Autodesk Inventor part; units mm, degrees
ref_plane "YZ Plane" through (0, 0, 0) normal (1, 0, 0) x (0, 1, 0)
ref_plane "XZ Plane" through (0, 0, 0) normal (0, 1, 0) x (-1, 0, 0)
ref_plane "XY Plane" through (0, 0, 0) normal (0, 0, 1) x (1, 0, 0)
sketch "Esboço1" plane through (0, 0, 0) normal (0, 0, 1) x (1, 0, 0)
  line L0 (0, 0) -> (110, 0)
  line L1 (110, 0) -> (110, 15)
  line L2 (110, 15) -> (0, 15)
  line L3 (0, 15) -> (0, 0)
  dimension "d0" = 110
  dimension "d1" = 15
extrude "Extrusão1" add sketch "Esboço1" along normal blind 15
chamfer "Chanfro1" distance 10 distance2 32 1 edges at (110, 15, 7.5) measured on face at (110, 5, 5)
sketch "Esboço2" plane through (0, 0, 0) normal (0, -1, 0) x (1, 0, 0)
  line L0 (0, 15) -> (110, 15)
  line L1 (0, 0) -> (0, 15)
  point P0 (13, 7.5)
  point P1 (66, 7.5)
  dimension "d7" = 7.5
  dimension "d8" = 13
  dimension "d25" = 53
hole "Furo1" at (13, 0, 7.5) at (66, 0, 7.5) direction (0, 1, 0) diameter 8.376 end through all
properties part number "Garra2"
Can you work these out from the model? Positions are in its coordinate system, mm. Coordinates: 2 decimals unless noted, no trailing zeros. Write each loop counter-clockwise with the first axis right and the second up, starting at its lowest first coordinate (ties: lowest second). Pieces come first, ordered by that corner, then holes.
Q1. If we mould it in two halves opening along Z, with no side actions, what happens to faces 1 (the face through (0, 8, 7)), 2 (the face through (70.088, 7.605, 8.408)), 3 (the face through (54, 8, 0))? For each: +Z half, -Z half, draft (parallel to the pull), parting line (faces both ways), or undercut.
Results found:
face 1: draft
face 2: undercut
face 3: -Z half
Q2. Imagine slicing it at C-C, the plane y = 11. List the corners of the cut face in (x, z) for me, plus the area to 3 significant figures.
Results found:
outline: (0, 0) - (90.8, 0) - (90.8, 15) - (0, 15) - close; hole circle Ø8.38 at (13, 7.5); hole circle Ø8.38 at (66, 7.5)
area: 1,250 mm2
Q3. Imagine slicing it at D-D, the plane x = 11. List the corners of the cut face in (y, z) for me.
Results found:
outline: (0, 0) - (15, 0) - (15, 3.82) - (0, 3.82) - close; (0, 11.18) - (15, 11.18) - (15, 15) - (0, 15) - close
Q4. Imagine slicing it at A-A, the plane z = 7.5. List the corners of the cut face in (x, y) for me, plus the area to 3 significant figures.
Results found:
outline: (0, 0) - (8.81, 0) - (8.81, 15) - (0, 15) - close; (17.19, 0) - (61.81, 0) - (61.81, 15) - (17.19, 15) - close; (70.19, 0) - (110, 0) - (110, 5) - (78, 15) - (70.19, 15) - close
area: 1,240 mm2
Q5. For P1, Ø6.5, axis at x = 66, z = 7.5, coming from the +Y side, with a flat end and sliding along its axis, tell me the tip position at first contact or that it passes through.
Results found:
P1: passes through
Q6. Imagine slicing it at B-B, the plane x = 66. List the corners of the cut face in (y, z) for me, plus the area to 3 significant figures.
Results found:
outline: (0, 0) - (15, 0) - (15, 3.31) - (0, 3.31) - close; (0, 11.69) - (15, 11.69) - (15, 15) - (0, 15) - close
area: 99.4 mm2
Q7. Please list where these lines run through material, in increasing order: L1, parallel to Z at x = 13, y = 7.5; L2, parallel to X at y = 1, z = 10.75; L3, parallel to X at y = 4, z = 4.5.
Results found:
L1: z = 0 to 3.31, 11.69 to 15
L2: x = 0 to 10.36, 15.64 to 63.36, 68.64 to 110
L3: x = 0 to 10.08, 15.92 to 63.08, 68.92 to 110
